from build123d import *

# Parameters (mm, degrees)
BOSS_EXTRUDE1_DEPTH = 44.7
SKETCH2_R           = 1.25
BOSS_EXTRUDE2_DEPTH = 4.1
SKETCH3_R           = 3.5
BOSS_EXTRUDE3_DEPTH = 2.1


with BuildPart() as part:
    # Sketch1 → Boss-Extrude1 (new body)
    with BuildSketch(Plane(origin=(0, 0, 0), x_dir=(1, 0, 0), z_dir=(0, 1, 0))):
        with BuildLine():
            Line((-10.5, 8), (10.5, 8))
            ThreePointArc((10.5, 8), (12.267766953, 7.267766953), (13, 5.5))
            Line((13, 5.5), (13, -5.5))
            ThreePointArc((13, -5.5), (12.267766953, -7.267766953), (10.5, -8))
            Line((10.5, -8), (-10.5, -8))
            ThreePointArc((-10.5, -8), (-12.267766953, -7.267766953), (-13, -5.5))
            Line((-13, -5.5), (-13, 5.5))
            ThreePointArc((-13, 5.5), (-12.267766953, 7.267766953), (-10.5, 8))
        make_face()
    extrude(amount=BOSS_EXTRUDE1_DEPTH)

    # Sketch2 → Boss-Extrude2 (add)
    with BuildSketch(Plane(origin=(0, 44.7, 0), x_dir=(1, 0, 0), z_dir=(0, 1, 0))):
        with Locations((-6.5, 0)):
            Circle(SKETCH2_R)
        with Locations((6.5, 0)):
            Circle(SKETCH2_R)
    extrude(amount=BOSS_EXTRUDE2_DEPTH)

    # Sketch3 → Boss-Extrude3 (add)
    with BuildSketch(Plane(origin=(0, 48.8, 0), x_dir=(1, 0, 0), z_dir=(0, 1, 0))):
        with Locations((-6.5, 0)):
            Circle(SKETCH3_R)
        with Locations((6.5, 0)):
            Circle(SKETCH3_R)
    extrude(amount=-BOSS_EXTRUDE3_DEPTH)


solid = part.part
Can you work these out from the model? Positions are in its coordinate system, mm. A direction names the side the tool comes from. Coordinates: 2 decimals unless noted, no trailing zeros. Write each loop counter-clockwise with the first axis right and the second up, starting at its lowest first coordinate (ties: lowest second). Pieces come first, ordered by that corner, then holes. Notation, with made-up numbers: (88, 9) - (98, 9) arc R12 cw to (98, 25) - close; hole circle Ø4 at (66, 83). An arc over 180 degrees is marked (long way). Return JSON: item names as keys, results as strings. Group by question number.
Item 1: Which directions (+Z, -Z, +X, -X, +Y, -Y) give clear straight access to the entire face, cutting with the end or side of a thin tool? Please do faces 1 (the face through (6, 46.7, 2)), 2 (the face through (-12.287, 22.037, -7.248)), 3 (the face through (8.115, 47.765, 3.105)).
Item 2: We'd pull the mould along Y, two halves only. Please class faces 4 (the face through (-7.75, 45.69, -0.05)), 5 (the face through (13, 22, 0)), 6 (the face through (5.25, 45.69, -0.05)), 7 (the face through (6, 48.8, 0)): pulls with the +Y half, pulls with the -Y half, needs draft (parallel to the pull), parting line crosses it, or undercut.
Item 3: I'm going to push flat-ended pins straight in: pin 1 Ø1.5 at (x, z) = (-10, 4.5) entering from +Y; pin 2 Ø5.5 at (x, z) = (-6, -1) entering from -Y. Where does each tip first touch, or does it pass through?
Item 4: If we section it at D-D (x = 2.5): Write out the boundary of the cut face in (y, z).
Item 5: If we section it at C-C (z = -7): Write out the boundary of the cut face in (x, y).
Item 6: Please list where these lines run through material, in increasing order: probe 1 along Y at (x, z) = (8.5, 0.5); probe 2 along Y at (x, z) = (10, 3.75); probe 3 along Z at (x, y) = (11, 23).
Item 7: If we section it at B-B (x = -6.5): Write out the boundary of the cut face in (y, z).
Item 8: If we section it at A-A (z = -2.75): Write out the boundary of the cut face in (x, y).
Return value:
{
 "1": {"face 1": "none", "face 2": "-Z, -X, +Y, -Y", "face 3": "+Y"},
 "2": {"face 4": "undercut", "face 5": "needs draft", "face 6": "undercut", "face 7": "pulls with the +Y half"},
 "3": {"pin 1": "stops at y = 44.7", "pin 2": "stops at y = 0"},
 "4": {"outline": "(0, -8) - (44.7, -8) - (44.7, 8) - (0, 8) - close"},
 "5": {"outline": "(-12.5, 0) - (12.5, 0) - (12.5, 44.7) - (-12.5, 44.7) - close"},
 "6": {"probe 1": "y = 0 to 44.7, 46.7 to 48.8", "probe 2": "y = 0 to 44.7", "probe 3": "z = -7.95 to 7.95"},
 "7": {"outline": "(0, -8) - (44.7, -8) - (44.7, -1.25) - (46.7, -1.25) - (46.7, -3.5) - (48.8, -3.5) - (48.8, 3.5) - (46.7, 3.5) - (46.7, 1.25) - (44.7, 1.25) - (44.7, 8) - (0, 8) - close"},
 "8": {"outline": "(-13, 0) - (13, 0) - (13, 44.7) - (-13, 44.7) - close; (-8.67, 46.7) - (-4.33, 46.7) - (-4.33, 48.8) - (-8.67, 48.8) - close; (4.33, 46.7) - (8.67, 46.7) - (8.67, 48.8) - (4.33, 48.8) - close"}
}
